from build123d import *

# Parameters (mm, degrees)
SKETCH13_W          = 69.282032303
SKETCH13_H          = 60
BOSS_EXTRUDE3_DEPTH = 80
CUT_EXTRUDE5_DEPTH  = 80
SKETCH15_R          = 12
CUT_EXTRUDE6_DEPTH  = 80


with BuildPart() as part:
    # Sketch13 → Boss-Extrude3 (new body)
    with BuildSketch(Plane(origin=(0, 0, 0), x_dir=(1, 0, 0), z_dir=(0, 1, 0))):
        with Locations((-34.641016152, -30)):
            Rectangle(SKETCH13_W, SKETCH13_H)
    extrude(amount=BOSS_EXTRUDE3_DEPTH)

    # Sketch14 → Cut-Extrude5 (cut)
    with BuildSketch(Plane(origin=(0, 0, 0), x_dir=(0, 0, -1), z_dir=(1, 0, 0))):
        Polygon((-60, 80), (0, 20), (0, 80), align=None)
    extrude(amount=-CUT_EXTRUDE5_DEPTH, mode=Mode.SUBTRACT)

    # Sketch15 → Cut-Extrude6 (cut)
    with BuildSketch(Plane(origin=(0, 0, 0), x_dir=(-1, 0, 0), z_dir=(0, -1, 0))):
        Polygon((69.282032303, -30), (51.961524227, -60), (69.282032303, -60), align=None)
        Polygon((51.961524227, 0), (69.282032303, -30), (69.282032303, 0), align=None)
        Polygon((0, -60), (17.320508076, -60), (0, -30), align=None)
        Polygon((0, 0), (0, -30), (17.320508076, 0), align=None)
        with Locations(Location((34.641016151, -30, 0), (0, 0, 90))):
            Circle(SKETCH15_R)
    extrude(amount=-CUT_EXTRUDE6_DEPTH, mode=Mode.SUBTRACT)


solid = part.part
Build history of the part. All positions in model axes, mm. Round coordinates to 2 decimals unless told otherwise and drop trailing zeros. Loops run counter-clockwise (first coordinate to the right, second up) from the corner with the lowest first, then second, coordinate; pieces in that order, holes last. Notation, with made-up numbers: (86.25, 9) -> (137.25, 9) arc R9 ccw to (137.25, 23) -> close; hole circle Ø3 at (-31.5, 9.25). An arc over 180 degrees is marked (long way). Answer in a Markdown table with one row per item.
Item 1: Mould opens along X. For faces 1 (the flat face through (-6.615, 19.094, 18.543)), 2 (the flat face through (-62.425, 19.094, 18.123)), 3 (the cylindrical face through (-34.11, 23.87, 41.99)), 4 (the flat face through (-35, 39, 60)) say: +X half, -X half, draft (parallel to the pull), parting line (faces both ways), or undercut.
Answers below:
| item | result |
|---|---|
| face 1 | +X half |
| face 2 | -X half |
| face 3 | undercut |
| face 4 | draft |
Item 2: Pin check, flat tips, straight feed: pin 1 (3 mm diameter, centred on x = -58.5, y = 35, fed in from -Z); pin 2 (10 mm diameter, centred on x = -10.5, y = 25.5, fed in from -Z); pin 3 (3 mm diameter, centred on x = -51, z = 23.5, fed in from +Y). Stop position of each tip, or through.
Answers below:
| item | result |
|---|---|
| pin 1 | stops at z = 13.5 |
| pin 2 | stops at z = 3.72 |
| pin 3 | stops at y = 45 |
Item 3: Saw through at D-D (x = -19.5). Write the cut outline in (y, z), and give its area (3 significant figures).
Answers below:
| item | result |
|---|---|
| outline | (0, 0) -> (20, 0) -> (80, 60) -> (0, 60) -> close |
| area | 3,000 mm² |
Item 4: Drill centre lines: L1, parallel to X at y = 24, z = 30; L2, parallel to Y at x = -11, z = 40; L3, parallel to Z at x = -27.5, y = 20.5. Where is each one in solid material? Low to high. Write a range as [from, to].
Answers below:
| item | result |
|---|---|
| L1 | x = [-69.28, -46.64], [-22.64, 0] |
| L2 | y = [0, 60] |
| L3 | z = [0.5, 20.36], [39.64, 60] |
Item 5: Saw through at A-A (z = 32). Write the cut outline in (x, y), and give its area (3 significant figures).
Answers below:
| item | result |
|---|---|
| outline | (-68.13, 0) -> (-46.47, 0) -> (-46.47, 52) -> (-68.13, 52) -> close; (-22.81, 0) -> (-1.15, 0) -> (-1.15, 52) -> (-22.81, 52) -> close |
| area | 2,250 mm² |
Item 6: Saw through at B-B (y = 26). Write the cut outline in (x, z).
Answers below:
| item | result |
|---|---|
| outline | (-69.28, 30) -> (-55.43, 6) -> (-13.86, 6) -> (0, 30) -> (-17.32, 60) -> (-51.96, 60) -> close; hole circle Ø24 at (-34.64, 30) |
Item 7: Saw through at C-C (x = -37). Write the cut outline in (y, z).
Answers below:
| item | result |
|---|---|
| outline | (0, 0) -> (20, 0) -> (38.23, 18.23) -> (0, 18.23) -> close; (0, 41.77) -> (61.77, 41.77) -> (80, 60) -> (0, 60) -> close |
